Geometry: final body of the model. Coordinates: model frame, mm. Round coordinates to 2 decimals unless told otherwise and drop trailing zeros. Write each loop counter-clockwise with the first axis right and the second up, starting at its lowest first coordinate (ties: lowest second). Pieces come first, ordered by that corner, then holes. Notation, with made-up numbers: M 42.25,77 L 62.25,77 A35 ccw 62.25,110 Z; hole C 52.5,43 d8. An arc over 180 degrees is marked long. Use one line per item in the form item = value. Start each with the question number.
Item 1: Section query C-C (z = 36.5). Return loops of the section in (x, y), and give its area (3 significant figures).
Item 2: Pin query (flat end, axial travel): pin 1 Ø4 at (x, z) = (-6.5, -4.5) entering from -Y; pin 2 Ø1.2 at (x, y) = (-5, -1.5) entering from +Z. Return the tip coordinate at first contact, or that it passes through.
Item 3: Section query A-A (x = -2.5). Return loops of the section in (y, z) (3 decimals).
Item 4: Section query D-D (x = -35.5). Return loops of the section in (y, z).
Item 5: Ray query, probe 1 along Z at (x, y) = (-35.5, -1.1); probe 2 along Z at (x, y) = (-34, -2.8); probe 3 along Z at (x, y) = (8.5, -1) (3 decimals). Return the intervals inside material, ascending.
Item 6: Section query B-B (y = -3.15). State how many separate pieces and enclosed holes the cut face has, and give its area (3 significant figures).
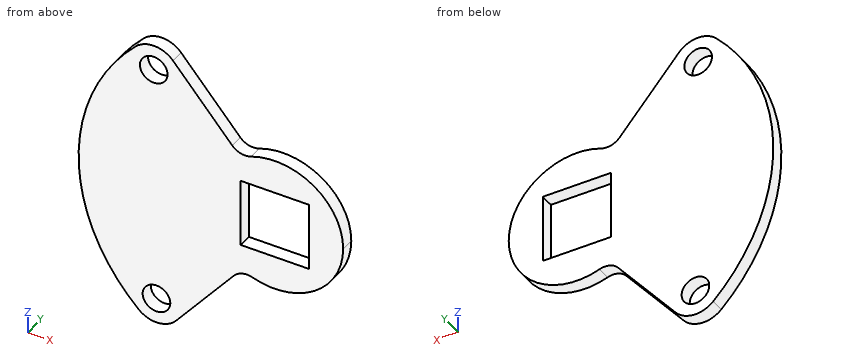
from build123d import *

# Parameters (mm, degrees)
F0_W     = 20.05
F0_H     = 20.05
F1_DEPTH = 4
F2_D     = 8.1
F3_R     = 5


with BuildPart() as f1:
    # F0 (on Front) → F1 (new body)
    with BuildSketch(Plane.XZ):
        with BuildLine():
            ThreePointArc((-9.6465038341, -17.519844856), (10.1752131014, -17.2181601323), (20, 0))
            ThreePointArc((20, 0), (9.9808325833, 17.331560257), (-10.0382980944, 17.2983401333))
            ThreePointArc((-10.0382980944, 17.2983401333), (-19.9987339156, -0.2250372661), (-9.6465038341, -17.519844856))
        make_face()
        Rectangle(F0_W, F0_H, mode=Mode.SUBTRACT)
        with BuildLine():
            ThreePointArc((-9.6465038341, -17.519844856), (-19.9987339156, -0.2250372661), (-10.0382980944, 17.2983401333))
            Line((-10.0382980944, 17.2983401333), (-29.8339876344, 40.1239726576))
            ThreePointArc((-29.8339876344, 40.1239726576), (-28.4734399333, 37.8325737503), (-28, 35.2100837829))
            ThreePointArc((-28, 35.2100837829), (-38.3559150153, 28.275118071), (-40.8249998468, 40.4915965048))
            ThreePointArc((-40.8249998468, 40.4915965048), (-57.4963600088, -0.6469820224), (-39.9035086306, -41.3999999875))
            ThreePointArc((-39.9035086306, -41.3999999875), (-37.6324685474, -29.09760762), (-27.1987031458, -36))
            ThreePointArc((-27.1987031458, -36), (-27.6430799913, -38.5432620593), (-28.9235516531, -40.785146313))
            Line((-28.9235516531, -40.785146313), (-9.6465038341, -17.519844856))
        make_face()
        with BuildLine():
            ThreePointArc((-28, 35.2100837829), (-28.4734399333, 37.8325737503), (-29.8339876344, 40.1239726576))
            ThreePointArc((-29.8339876344, 40.1239726576), (-35.2492826138, 42.7058919977), (-40.8249998468, 40.4915965048))
            ThreePointArc((-40.8249998468, 40.4915965048), (-38.3559150153, 28.275118071), (-28, 35.2100837829))
        make_face()
        with BuildLine():
            ThreePointArc((-39.9035086306, -41.3999999875), (-34.2793764206, -43.488268498), (-28.9235516531, -40.785146313))
            ThreePointArc((-28.9235516531, -40.785146313), (-27.6430799913, -38.5432620593), (-27.1987031458, -36))
            ThreePointArc((-27.1987031458, -36), (-37.6324685474, -29.09760762), (-39.9035086306, -41.3999999875))
        make_face()
    extrude(amount=F1_DEPTH)

    # F2 (through all)
    with Locations(Plane(origin=(0, 0, 0), x_dir=(1, 0, 0), z_dir=(0, 1, 0))):
        with Locations((-34.6987031458, 36), (-35.5, -35.2100837829)):
            Hole(F2_D / 2)

    # F3
    f3_edges = [f1.edges().sort_by_distance(p)[0] for p in [
        (-10.038298, -2, 17.29834),
        (-9.646504, -2, -17.519845),
    ]]
    fillet(f3_edges, radius=F3_R)


solid = f1.part
Working result:
q1.outline = M -44.43,-4 L -39.34,-4 L -39.34,0 L -44.43,0 Z; M -31.66,-4 L -26.69,-4 L -26.69,0 L -31.66,0 Z
q1.area = 40.2 mm²
q2.pin_1 = through
q2.pin_2 = 19.51
q3.outline = M -4,-19.843 L 0,-19.843 L 0,-10.025 L -4,-10.025 Z; M -4,10.025 L 0,10.025 L 0,19.843 L -4,19.843 Z
q4.outline = M -4,-43.46 L 0,-43.46 L 0,-39.97 L -4,-39.97 Z; M -4,-32.03 L 0,-32.03 L 0,31.16 L -4,31.16 Z; M -4,39.26 L 0,39.26 L 0,42.71 L -4,42.71 Z
q5.probe_1 = -43.46 to -39.97, -32.03 to 31.16, 39.26 to 42.71
q5.probe_2 = -43.47 to -39.99, -32.01 to 31.45, 38.97 to 42.56
q5.probe_3 = -18.104 to -10.025, 10.025 to 18.104
q6.separate_pieces = 1
q6.enclosed_holes = 3
q6.area = 3,530 mm²
